Source: CAD feature listing. Evaluate the final solid. Frame: model axes, mm. Coordinates: 2 decimals unless noted, no trailing zeros. Loops run counter-clockwise (first coordinate to the right, second up) from the corner with the lowest first, then second, coordinate; pieces in that order, holes last. Notation, with made-up numbers: (79, -30) - (114, -30) arc R23 ccw to (114, -8) - close; hole circle Ø10 at (77, 89.25). An arc over 180 degrees is marked (long way). Write item = value, one per line. Start each with the question number.
from build123d import *

# Parameters (mm, degrees)
SKETCH_6441_R           = 1.55
SKETCH_6441_R_2         = 2.75
EXTRUDE_13625_DEPTH     = 2
FILLET_13791_R          = 5
SKETCH_13989_W          = 15.5
SKETCH_13989_H          = 2.5
CUT_EXTRUDE_14254_DEPTH = 246.566929957
SKETCH_14301_R          = 1.55
CUT_EXTRUDE_14313_DEPTH = 246.566929957
SKETCH_14441_R          = 0.5
CUT_EXTRUDE_14789_DEPTH = 246.566929957


with BuildPart() as part:
    # Sketch 6441 → Extrude 13625 (new body)
    with BuildSketch(Plane.XY):
        with BuildLine():
            Line((136.084964988, 154.573657256), (183.657608305, 107.001013939))
            Line((183.657608305, 107.001013939), (181.978644035, 42.883955268))
            Line((181.978644035, 42.883955268), (163.126615581, 12.12024083))
            Line((163.126615581, 12.12024083), (163.126615581, -12.12024083))
            Line((163.126615581, -12.12024083), (182.978644035, -44.515806956))
            Line((182.978644035, -44.515806956), (182.978644035, -110.861958724))
            Line((182.978644035, -110.861958724), (136.031615851, -157.808986908))
            Line((136.031615851, -157.808986908), (48.416521639, -157.808986908))
            Line((48.416521639, -157.808986908), (21.353443149, -156.6))
            Line((21.353443149, -156.6), (17.45, -156.6))
            Line((17.45, -156.6), (17.45, -154.5))
            Line((17.45, -154.5), (16.1, -154.5))
            Line((16.1, -154.5), (16.1, -146))
            Line((16.1, -146), (12, -146))
            Line((12, -146), (12, -163))
            Line((12, -163), (7.5, -163))
            Line((7.5, -163), (3.358391833, -150.5))
            Line((3.358391833, -150.5), (0.25, -150.5))
            Line((0.25, -150.5), (0.25, -133.5))
            Line((0.25, -133.5), (7.25, -133.5))
            Line((7.25, -133.5), (12.591750717, -128.153933031))
            Line((12.591750717, -128.153933031), (24.501126091, -128.153933031))
            Line((24.501126091, -128.153933031), (24.501126091, -130.1))
            Line((24.501126091, -130.1), (26.001126091, -130.1))
            Line((26.001126091, -130.1), (26.001126091, -139.07316335))
            Line((26.001126091, -139.07316335), (48.416521639, -143.308986908))
            Line((48.416521639, -143.308986908), (86.829107225, -143.308986908))
            ThreePointArc((86.829107225, -143.308986908), (160.06208789, -116.291913973), (163.126615581, -38.294475829))
            Line((163.126615581, -38.294475829), (152.626615581, -21.160033114))
            Line((152.626615581, -21.160033114), (152.626615581, -3.75))
            Line((152.626615581, -3.75), (153.876615581, -2.5))
            Line((153.876615581, -2.5), (153.876615581, 2.5))
            Line((153.876615581, 2.5), (152.626615581, 3.75))
            Line((152.626615581, 3.75), (152.626615581, 21.160033114))
            Line((152.626615581, 21.160033114), (163.126615581, 38.294475829))
            ThreePointArc((163.126615581, 38.294475829), (161.123508786, 114.790038144), (90.426598369, 144.073657256))
            Line((90.426598369, 144.073657256), (58.529829123, 144.43553015))
            Line((58.529829123, 144.43553015), (48.416521639, 134.322222666))
            Line((48.416521639, 134.322222666), (48.416521639, 120.077827626))
            Line((48.416521639, 120.077827626), (42.916521639, 115.25))
            Line((42.916521639, 115.25), (34.629076425, 115.25))
            ThreePointArc((34.629076425, 115.25), (34.835, 129.535814466), (33.42537009, 143.753403677))
            ThreePointArc((33.42537009, 143.753403677), (33.93663348, 146.980087891), (36.239566526, 149.297280299))
            Line((36.239566526, 149.297280299), (45.830022829, 154.240299961))
            ThreePointArc((45.830022829, 154.240299961), (46.497305667, 154.48912704), (47.204437863, 154.573657256))
            Line((47.204437863, 154.573657256), (136.084964988, 154.573657256))
        make_face()
        with Locations((39.335, 139.4323004)):
            Circle(SKETCH_6441_R, mode=Mode.SUBTRACT)
        with Locations((39.335, 129.0823004)):
            Circle(SKETCH_6441_R_2, mode=Mode.SUBTRACT)
        with Locations((39.335, 120.1823004)):
            Circle(SKETCH_6441_R, mode=Mode.SUBTRACT)
        with Locations((14.6, -133.5)):
            Circle(SKETCH_6441_R, mode=Mode.SUBTRACT)
        with Locations((22.35, -133.5)):
            Circle(SKETCH_6441_R, mode=Mode.SUBTRACT)
    extrude(amount=EXTRUDE_13625_DEPTH)

    # Fillet 13791
    fillet_13791_edges = [part.edges().sort_by_distance(p)[0] for p in [
        (90.426598369, 144.073657256, 1),
        (48.416521639, 120.077827626, 1),
        (86.829107225, -143.308986908, 1),
    ]]
    fillet(fillet_13791_edges, radius=FILLET_13791_R)

    # Sketch 13989 → Cut-Extrude 14254 (cut, through all)
    with BuildSketch(Plane.XY):
        Polygon((149.075304921, -134.865802902), (160.035460029, -123.905647794), (161.803226982, -125.673414746), (150.843071874, -136.633569855), align=None)
        with Locations((68.468496842, -151.058986908)):
            Rectangle(SKETCH_13989_W, SKETCH_13989_H)
        with Locations((101.468496842, -151.058986908)):
            Rectangle(SKETCH_13989_W, SKETCH_13989_H)
    extrude(amount=CUT_EXTRUDE_14254_DEPTH, mode=Mode.SUBTRACT)

    # Sketch 14301 → Cut-Extrude 14313 (cut, through all)
    with BuildSketch(Plane.XY):
        with Locations((157.876615581, 0)):
            Circle(SKETCH_14301_R)
        with Locations((174.201788477, -107.226466117)):
            Circle(SKETCH_14301_R)
        with Locations((123.531615851, -151.058986908)):
            Circle(SKETCH_14301_R)
        with Locations((174.880752746, 103.365521332)):
            Circle(SKETCH_14301_R)
        with Locations((132.832155813, 146.72068123)):
            Circle(SKETCH_14301_R)
        with Locations((174.201788477, -46.867558315)):
            Circle(SKETCH_14301_R)
        with Locations((174.787496024, 45.014070354)):
            Circle(SKETCH_14301_R)
    extrude(amount=CUT_EXTRUDE_14313_DEPTH, mode=Mode.SUBTRACT)

    # Sketch 14441 → Cut-Extrude 14789 (cut, through all)
    with BuildSketch(Plane.XY):
        with Locations((60.718496842, -149.808986908)):
            Circle(SKETCH_14441_R)
        with Locations((60.718496842, -152.308986908)):
            Circle(SKETCH_14441_R)
        with Locations((76.218496842, -152.308986908)):
            Circle(SKETCH_14441_R)
        with Locations((76.218496842, -149.808986908)):
            Circle(SKETCH_14441_R)
        with Locations((93.718496842, -149.808986908)):
            Circle(SKETCH_14441_R)
        with Locations((93.718496842, -152.308986908)):
            Circle(SKETCH_14441_R)
        with Locations((109.218496842, -152.308986908)):
            Circle(SKETCH_14441_R)
        with Locations((109.218496842, -149.808986908)):
            Circle(SKETCH_14441_R)
        with Locations((149.075304921, -134.865802902)):
            Circle(SKETCH_14441_R)
        with Locations((150.843071874, -136.633569855)):
            Circle(SKETCH_14441_R)
        with Locations((160.035460029, -123.905647794)):
            Circle(SKETCH_14441_R)
        with Locations((161.803226982, -125.673414746)):
            Circle(SKETCH_14441_R)
        with Locations((12, -146)):
            Circle(SKETCH_14441_R)
        with Locations((16.1, -146)):
            Circle(SKETCH_14441_R)
        with Locations((17.45, -154.5)):
            Circle(SKETCH_14441_R)
        with Locations((24.501126091, -130.1)):
            Circle(SKETCH_14441_R)
    extrude(amount=CUT_EXTRUDE_14789_DEPTH, mode=Mode.SUBTRACT)


solid = part.part
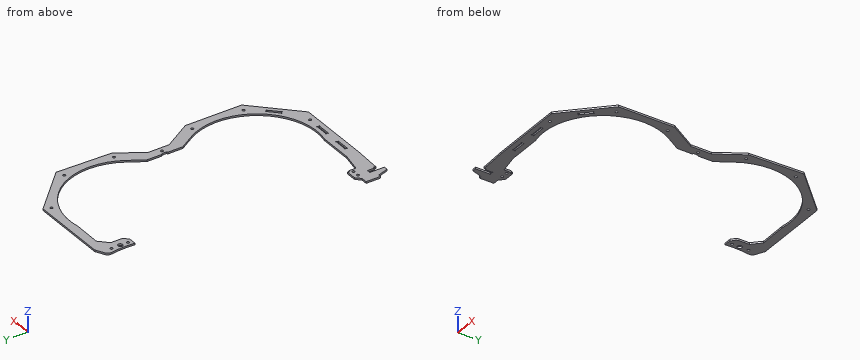
Item 1: Cut plane A-A (x = 169). Return the cut outline in (y, z), then the cut area to 3 significant figures.
Item 2: Cut plane C-C (z = 0.55). State how many separate pieces and enclosed holes the cut face has, then the cut area to 3 significant figures.
Item 3: First-contact query: pin 1 (0.5 mm diameter, centred on y = -156, z = 1, fed in from -X); pin 2 (8 mm diameter, centred on x = 47, y = 109, fed in from +Z); pin 3 (0.6 mm diameter, centred on y = -155.5, z = 0.5, fed in from +X); pin 4 (0.6 mm diameter, centred on y = 15, z = 1, fed in from -X). Flat tips, straight axial feed; report the tip coordinate or a pass-through.
Item 4: Cut plane D-D (y = -95.5). Return the cut outline in (x, z).
Item 5: Material intervals for L1, parallel to Y at x = 63, z = 0.6; L2, parallel to Y at x = 85, z = 0.85; L3, parallel to Y at x = 160, z = 0.2, sorted ascending. Write a range as [from, to].
Item 6: Cut plane B-B (x = 103). Return the cut outline in (y, z), then the cut area to 3 significant figures.
Responses:
q1.outline = (-124.84, 0) - (-99.68, 0) - (-99.68, 2) - (-124.84, 2) - close; (-50.32, 0) - (-21.7, 0) - (-21.7, 2) - (-50.32, 2) - close; (21.7, 0) - (50.32, 0) - (50.32, 2) - (21.7, 2) - close; (99.68, 0) - (121.66, 0) - (121.66, 2) - (99.68, 2) - close
q1.area = 209 mm2
q2.separate_pieces = 1
q2.enclosed_holes = 15
q2.area = 7,590 mm2
q3.pin_1 = 5.1
q3.pin_2 = through
q3.pin_3 = 138.64
q3.pin_4 = 152.63
q4.outline = (170.42, 0) - (182.98, 0) - (182.98, 2) - (170.42, 2) - close
q5.L1 = [-157.81, -152.31], [-149.81, -143.31], [144.38, 154.57]
q5.L2 = [-157.81, -143.31], [144.14, 154.57]
q5.L3 = [-133.84, -127.48], [-123.41, -116.38], [-33.19, 33.19], [116.38, 130.66]
q6.outline = (-157.81, 0) - (-152.31, 0) - (-152.31, 2) - (-157.81, 2) - close; (-149.81, 0) - (-145.25, 0) - (-145.25, 2) - (-149.81, 2) - close; (145.25, 0) - (154.57, 0) - (154.57, 2) - (145.25, 2) - close
q6.area = 38.8 mm2
